Part model, mm, in its own coordinate system. A direction names the side the tool comes from. Give positions to 0.01 mm unless a question says otherwise; leave off trailing zeros. Write each loop counter-clockwise with the first axis right and the second up, starting at its lowest first coordinate (ties: lowest second). Pieces come first, ordered by that corner, then holes. Notation, with made-up numbers: M 33.5,51 L 64.5,51 A26 cw 64.5,77 Z; hole C 2,27 d1. An arc over 180 degrees is marked long. Answer as CSV lines item,"result". Start each with the question number.
Item 1: Wall check: L1, parallel to X at y = 6.5, z = -11.5 (3 decimals); L2, parallel to X at y = -8.95, z = -25.4 (3 decimals). Give the ranges that are in metal, low to high. Write a range as from..to.
Item 2: Band-saw the part on A-A, the plane y = 7.5. List the corners of the cut face in (x, z) (3 decimals).
Item 3: Two-plate mould, pull along Z, no slides. Class faces 1 (the flat face through (-1, -9, 60)), 2 (the flat face through (-6, 8.625, 1)), 3 (the cylindrical face through (-9.069, -0.521, -44.034)): +Z half, -Z half, draft (parallel to the pull), parting line (faces both ways), or undercut.
Item 4: Band-saw the part on C-C, the plane z = -39. List the corners of the cut face in (x, y) (3 decimals), then the cut area to 3 significant figures.
Item 5: 3-axis set-ups, long thin cutter, end or side, ignore diameter. For faces 4 (the flat face through (-8.625, 0, 1)), 5 (the flat face through (-1, -9, -60)): which of +Z, -Z, +X, -X, +Y, -Y reach the whole face in a straight line?
Item 6: Pin check, flat tip, straight feed: pin 1 (5 mm diameter, centred on y = 0, z = -48, fed in from +X). Stop position of the tip, or through.
Item 7: Band-saw the part on D-D, the plane y = 0. List the corners of the cut face in (x, z) (3 decimals), then the cut area to 3 significant figures.
from build123d import *

# Parameters (mm, degrees)
SKETCH1_W           = 19.05
SKETCH1_H           = 19.05
SKETCH1_W_2         = 17.25
SKETCH1_H_2         = 17.25
EXTRUDE_THIN1_DEPTH = 60
SKETCH2_R           = 4
CUT_EXTRUDE1_DEPTH  = 64.668109168
SKETCH3_R           = 4
CUT_EXTRUDE2_DEPTH  = 64.668109168


with BuildPart() as part:
    # Sketch1 → Extrude-Thin1 (new, symmetric)
    with BuildSketch(Plane.XY):
        Rectangle(SKETCH1_W, SKETCH1_H)
        Rectangle(SKETCH1_W_2, SKETCH1_H_2, mode=Mode.SUBTRACT)
    extrude(amount=EXTRUDE_THIN1_DEPTH, both=True)

    # Sketch2 → Cut-Extrude1 (cut, through all)
    with BuildSketch(Plane(origin=(9.525, 0, 0), x_dir=(0, 0, -1), z_dir=(1, 0, 0))):
        with Locations(Location((-48, 0, 0), (0, 0, 90))):
            Circle(SKETCH2_R)
        with Locations(Location((48, 0, 0), (0, 0, 90))):
            Circle(SKETCH2_R)
    extrude(amount=-CUT_EXTRUDE1_DEPTH, mode=Mode.SUBTRACT)

    # Sketch3 → Cut-Extrude2 (cut, through all)
    with BuildSketch(Plane(origin=(0, 9.525, 0), x_dir=(1, 0, 0), z_dir=(0, 1, 0))):
        with Locations(Location((0, -25.4, 0), (0, 0, 270))):
            Circle(SKETCH3_R)
        with Locations(Location((0, 25.4, 0), (0, 0, 270))):
            Circle(SKETCH3_R)
        with Locations(Location((0, 0, 0), (0, 0, 270))):
            Circle(SKETCH3_R)
    extrude(amount=-CUT_EXTRUDE2_DEPTH, mode=Mode.SUBTRACT)


solid = part.part
Output:
1,L1,"-9.525..-8.625, 8.625..9.525"
1,L2,"-9.525..-4, 4..9.525"
2,outline,"M -9.525,-60 L -8.625,-60 L -8.625,60 L -9.525,60 Z; M 8.625,-60 L 9.525,-60 L 9.525,60 L 8.625,60 Z"
3,face 1,"+Z half"
3,face 2,"draft"
3,face 3,"undercut"
4,outline,"M -9.525,-9.525 L 9.525,-9.525 L 9.525,9.525 L -9.525,9.525 Z; hole M -8.625,-8.625 L 8.625,-8.625 L 8.625,8.625 L -8.625,8.625 Z"
4,area,"65.3 mm²"
5,face 4,"+Z, -Z"
5,face 5,"-Z, +X, -X, +Y, -Y"
6,pin 1,"through"
7,outline,"M -9.525,-60 L -8.625,-60 L -8.625,-52 L -9.525,-52 Z; M -9.525,-44 L -8.625,-44 L -8.625,44 L -9.525,44 Z; M -9.525,52 L -8.625,52 L -8.625,60 L -9.525,60 Z; M 8.625,-60 L 9.525,-60 L 9.525,-52 L 8.625,-52 Z; M 8.625,-44 L 9.525,-44 L 9.525,44 L 8.625,44 Z; M 8.625,52 L 9.525,52 L 9.525,60 L 8.625,60 Z"
7,area,"187 mm²"
